Work out the finished part from the listing and answer in its coordinate system (mm). Face numbers are marked on the shaded views. A direction names the side the tool comes from. Round coordinates to 2 decimals unless told otherwise and drop trailing zeros. Loops run counter-clockwise (first coordinate to the right, second up) from the corner with the lowest first, then second, coordinate; pieces in that order, holes last.
```python
from build123d import *

# Parameters (mm, degrees)
F1_W      = 9
F1_H      = 83
F2_DEPTH  = 63
F3_R      = 2.85
F4_DEPTH  = 3.5
F5_R      = 1.6
F6_DEPTH  = 25
F7_W      = 40
F7_H      = 10
F8_DEPTH  = 40.2
F9_W      = 4.8
F9_H      = 40
F10_DEPTH = 2
F11_SIZE  = 1.8
F12_R     = 1.6
F13_DEPTH = 25
F14_W     = 4.8
F14_H     = 40
F15_DEPTH = 2
F16_SIZE  = 1.8
F17_R     = 1.6
F18_DEPTH = 25
F19_R     = 2.85
F20_DEPTH = 3.5
F21_R     = 2.85
F22_DEPTH = 3.5
F23_R     = 1.5
F24_DEPTH = 10


with BuildPart() as f2:
    # F1 (on Top) → F2 (new body)
    with BuildSketch(Plane.XY):
        with Locations((4.5, 41.5)):
            Rectangle(F1_W, F1_H)
    extrude(amount=F2_DEPTH)

    # F3 (on face) → F4 (cut)
    with BuildSketch(Plane.YZ.offset(9)):
        with Locations((8.5, 40.5)):
            Circle(F3_R)
        with Locations((8.5, 22.5)):
            Circle(F3_R)
        with Locations((76.5, 56.5)):
            Circle(F3_R)
        with Locations((76.5, 38.5)):
            Circle(F3_R)
        with Locations((76.5, 24.5)):
            Circle(F3_R)
        with Locations((76.5, 6.5)):
            Circle(F3_R)
    extrude(amount=-F4_DEPTH, mode=Mode.SUBTRACT)

    # F5 (on face) → F6 (cut)
    with BuildSketch(Plane.YZ.offset(9)):
        with Locations((8.5, 40.5)):
            Circle(F5_R)
        with Locations((8.5, 22.5)):
            Circle(F5_R)
        with Locations((76.5, 24.5)):
            Circle(F5_R)
        with Locations((76.5, 38.5)):
            Circle(F5_R)
        with Locations((76.5, 56.5)):
            Circle(F5_R)
        with Locations((76.5, 6.5)):
            Circle(F5_R)
    extrude(amount=-F6_DEPTH, mode=Mode.SUBTRACT)

    # F7 (on face) → F8 (join)
    with BuildSketch(Plane.YZ.offset(9)):
        with Locations((43, 16.4)):
            Rectangle(F7_W, F7_H)
        with Locations((43, 46.6)):
            Rectangle(F7_W, F7_H)
    extrude(amount=F8_DEPTH)

    # F9 (on face) → F10 (join)
    with BuildSketch(Plane(origin=(0, 0, 41.6), x_dir=(1, 0, 0), z_dir=(0, 0, -1))):
        with Locations((19.1, -43)):
            Rectangle(F9_W, F9_H)
        with Locations((39.1, -43)):
            Rectangle(F9_W, F9_H)
    extrude(amount=F10_DEPTH)

    # F11
    f11_edges = [f2.edges().sort_by_distance(p)[0] for p in [
        (21.5, 43, 39.6),
        (16.7, 43, 39.6),
        (41.5, 43, 39.6),
        (36.7, 43, 39.6),
    ]]
    chamfer(f11_edges, length=F11_SIZE)

    # F12 (on face) → F13 (cut)
    with BuildSketch(Plane(origin=(0, 0, 39.6), x_dir=(1, 0, 0), z_dir=(0, 0, -1))):
        with Locations((19.1, -33)):
            Circle(F12_R)
        with Locations((19.1, -53)):
            Circle(F12_R)
        with Locations((39.1, -33)):
            Circle(F12_R)
        with Locations((39.1, -53)):
            Circle(F12_R)
    extrude(amount=-F13_DEPTH, mode=Mode.SUBTRACT)

    # F14 (on face) → F15 (join)
    with BuildSketch(Plane.XY.offset(21.4)):
        with Locations((19.1, 43)):
            Rectangle(F14_W, F14_H)
        with Locations((39.1, 43)):
            Rectangle(F14_W, F14_H)
    extrude(amount=F15_DEPTH)

    # F16
    f16_edges = [f2.edges().sort_by_distance(p)[0] for p in [
        (21.5, 43, 23.4),
        (16.7, 43, 23.4),
        (36.7, 43, 23.4),
        (41.5, 43, 23.4),
    ]]
    chamfer(f16_edges, length=F16_SIZE)

    # F17 (on face) → F18 (cut)
    with BuildSketch(Plane.XY.offset(23.4)):
        with Locations((19.1, 33)):
            Circle(F17_R)
        with Locations((19.1, 53)):
            Circle(F17_R)
        with Locations((39.1, 33)):
            Circle(F17_R)
        with Locations((39.1, 53)):
            Circle(F17_R)
    extrude(amount=-F18_DEPTH, mode=Mode.SUBTRACT)

    # F19 (on face) → F20 (cut)
    with BuildSketch(Plane(origin=(0, 0, 11.4), x_dir=(1, 0, 0), z_dir=(0, 0, -1))):
        with Locations((19.1, -33)):
            Circle(F19_R)
        with Locations((19.1, -53)):
            Circle(F19_R)
        with Locations((39.1, -33)):
            Circle(F19_R)
        with Locations((39.1, -53)):
            Circle(F19_R)
    extrude(amount=-F20_DEPTH, mode=Mode.SUBTRACT)

    # F21 (on face) → F22 (cut)
    with BuildSketch(Plane.XY.offset(51.6)):
        with Locations((19.1, 53)):
            Circle(F21_R)
        with Locations((19.1, 33)):
            Circle(F21_R)
        with Locations((39.1, 53)):
            Circle(F21_R)
        with Locations((39.1, 33)):
            Circle(F21_R)
    extrude(amount=-F22_DEPTH, mode=Mode.SUBTRACT)

    # F23 (on face) → F24 (cut)
    with BuildSketch(Plane.YZ.offset(49.2)):
        with Locations((56.5, 16.4)):
            Circle(F23_R)
        with Locations((29.5, 16.4)):
            Circle(F23_R)
        with Locations((29.5, 46.6)):
            Circle(F23_R)
        with Locations((56.5, 46.6)):
            Circle(F23_R)
    extrude(amount=-F24_DEPTH, mode=Mode.SUBTRACT)


solid = f2.part
```
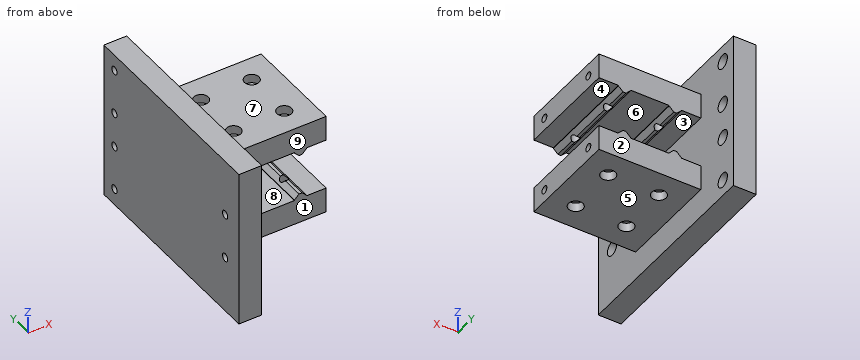
1. Determine the mould class of the marked faces 6, 7, 8 and 9 for opening direction Z: +Z half, -Z half, draft (parallel to the pull), parting line (faces both ways), or undercut.
Answer key:
face 6: undercut
face 7: +Z half
face 8: undercut
face 9: draft
2. Which of the six approach directions +Z, -Z, +X, -X, +Y, -Y give full straight-line access (tool end or side, diameter ignored) to the marked faces 1, 2, 3, 4 and 5?
Answer key:
face 1: +Z, -Z, +X, -Y
face 2: +Z, -Z, +X, +Y
face 3: +Y, -Y
face 4: +X, +Y, -Y
face 5: -Z, +X, +Y, -Y
3. Find section C-C (z = 13.5). Write down the section's boundary in (x, y).
Answer key:
outline: (0, 0) - (9, 0) - (9, 23) - (49.2, 23) - (49.2, 63) - (9, 63) - (9, 83) - (0, 83) - close; hole circle Ø5.7 at (19.1, 33); hole circle Ø5.7 at (19.1, 53); hole circle Ø5.7 at (39.1, 33); hole circle Ø5.7 at (39.1, 53)
4. Find section D-D (x = 28.5). Write down the section's boundary in (y, z).
Answer key:
outline: (23, 11.4) - (63, 11.4) - (63, 21.4) - (23, 21.4) - close; (23, 41.6) - (63, 41.6) - (63, 51.6) - (23, 51.6) - close
5. Consider probe 1 along Z at (x, y) = (6.7, 76.5); probe 2 along Z at (x, y) = (43, 56.5); probe 3 along Y at (x, z) = (39.1, 18). Determine where each line is inside the solid, lowest interval first.
Answer key:
probe 1: z = 0 to 3.65, 9.35 to 21.65, 27.35 to 35.65, 41.35 to 53.65, 59.35 to 63
probe 2: z = 11.4 to 14.9, 17.9 to 21.4, 41.6 to 45.1, 48.1 to 51.6
probe 3: y = 23 to 31.4, 34.6 to 51.4, 54.6 to 63
6. Find section A-A (y = 8.5). Write down the section's boundary in (x, z), then the cut area to 3 significant figures.
Answer key:
outline: (0, 0) - (9, 0) - (9, 19.65) - (5.5, 19.65) - (5.5, 20.9) - (0, 20.9) - close; (0, 24.1) - (5.5, 24.1) - (5.5, 25.35) - (9, 25.35) - (9, 37.65) - (5.5, 37.65) - (5.5, 38.9) - (0, 38.9) - close; (0, 42.1) - (5.5, 42.1) - (5.5, 43.35) - (9, 43.35) - (9, 63) - (0, 63) - close
area: 492 mm2
7. Given pin 1 (3 mm diameter, centred on x = 40.5, y = 34.5, fed in from +Z); pin 2 (4.5 mm diameter, centred on x = 19, y = 32.5, fed in from +Z); pin 3 (6 mm diameter, centred on y = 13, z = 34.5, fed in from +X), each flat-ended and moving along its own axis, determine where each tip first touches the part or whether it passes through.
Answer key:
pin 1: stops at z = 51.6
pin 2: stops at z = 48.1
pin 3: stops at x = 9
8. Find section B-B (z = 6.5). Write down the section's boundary in (x, y), then the cut area to 3 significant figures.
Answer key:
outline: (0, 0) - (9, 0) - (9, 73.65) - (5.5, 73.65) - (5.5, 74.9) - (0, 74.9) - close; (0, 78.1) - (5.5, 78.1) - (5.5, 79.35) - (9, 79.35) - (9, 83) - (0, 83) - close
area: 709 mm2
